Autodesk Inventor part; units mm, degrees
ref_plane "YZ Plane" through (0, 0, 0) normal (1, 0, 0) x (0, 1, 0)
ref_plane "XZ Plane" through (0, 0, 0) normal (0, 1, 0) x (-1, 0, 0)
ref_plane "XY Plane" through (0, 0, 0) normal (0, 0, 1) x (1, 0, 0)
sketch "Sketch2" plane through (0, 0, 0) normal (0, 0, 1) x (1, 0, 0)
  line L0 (0, 0) -> (2, 0)
  line L1 (2, 0) -> (2, 48.75)
  line L2 (2, 48.75) -> (0, 48.75)
  line L3 (0, 48.75) -> (0, 0)
  line L4 (2, 1) -> (1.75, 1)
  line L5 (1.75, 1) -> (1.75, 1.5)
  line L6 (1.75, 1.5) -> (2, 1.5)
  line L7 (2, 1.5) -> (2, 1)
  line L8 (2, 16) -> (1.75, 16)
  line L9 (1.75, 16) -> (1.75, 16.5)
  line L10 (1.75, 16.5) -> (2, 16.5)
  line L11 (2, 16.5) -> (2, 16)
  dimension "d3" = 2
  dimension "d4" = 48.75
  dimension "d5" = 1
  dimension "d6" = 0.5
  dimension "d7" = 0.25
  dimension "d8" = 16
  dimension "d9" = 0.5
  dimension "d10" = 0.25
revolve "Revolution1" add sketch "Sketch2" angle 360 about axis through (0, 48.75, 0) along (0, -1, 0) contours L3 L2 L1 L10 L9 L8 L6 L5 L4 L0
chamfer "Chamfer1" distance 0.25 angle 45 2 edges at (-2, 48.75, 0) (-2, 0, 0)
properties part number "SHAFT"
Build history of the part. All positions in model axes, mm. Give positions to 0.01 mm unless a question says otherwise; leave off trailing zeros. Order: outer loops, then holes, each group sorted by start corner. A loop starts at its lowest first (then second) coordinate and runs counter-clockwise, first axis right, second up. Notation, with made-up numbers: M 89,62 L 93,62 A24 cw 93,100 Z; hole C 19.25,-16.5 d1. An arc over 180 degrees is marked long. Put each result on its own line as item: value.
Item 1: Flat gauge pins, fed straight in: pin 1 Ø1 at (x, y) = (1, 21) entering from -Z; pin 2 Ø2 at (y, z) = (10.5, 1.5) entering from -X. Where does each tip first touch, or does it go through?
From the geometry:
pin 1: stops at z = -1.94
pin 2: stops at x = -1.94
Item 2: Slice it at A-A, the plane y = 37.5. Write the cut outline in (x, z).
From the geometry:
outline: C 0,0 d4
Item 3: Probe line 1 (Y direction, x = -0.65, z = -1.8); line 2 (Y direction, x = 1, z = 1.5); line 3 (Z direction, x = 0.95, y = 41). List the from-to ranges inside material, lowest first. Write a range as [from, to].
From the geometry:
line 1: y = [0.16, 1], [1.5, 16], [16.5, 48.59]
line 2: y = [0.05, 1], [1.5, 16], [16.5, 48.7]
line 3: z = [-1.76, 1.76]
Item 4: Two-plate mould, pull along Y, no slides. Class faces 1 (the cylindrical face through (0, 33, 2)), 2 (the cylindrical face through (1.617, 1.254, 0.67)), 3 (the cylindrical face through (1.617, 16.253, 0.67)), 4 (the flat face through (0, 48.75, 0)): +Y half, -Y half, draft (parallel to the pull), parting line (faces both ways), or undercut.
From the geometry:
face 1: draft
face 2: undercut
face 3: undercut
face 4: +Y half
